Verification items for the finished model (mm, model axes). Face numbers are marked on the shaded views. Round coordinates to 2 decimals unless told otherwise and drop trailing zeros. Order: outer loops, then holes, each group sorted by start corner. A loop starts at its lowest first (then second) coordinate and runs counter-clockwise, first axis right, second up. Notation, with made-up numbers: M 29,73.5 L 76,73.5 A16 cw 76,103.5 Z; hole C -9.75,80 d1. An arc over 180 degrees is marked long. Use one line per item in the form item = value. Start each with the question number.
Item 1: Thickness scan on probe 1 along X at (y, z) = (3.6, 21); probe 2 along Y at (x, z) = (8, 19); probe 3 along X at (y, z) = (2.3, 6.5). Record the ranges inside material, lowest first. Write a range as [from, to].
Item 2: Release check for a two-part mould opening along X. For the marked faces 1, 2 and 3 record: +X half, -X half, draft (parallel to the pull), parting line (faces both ways), or undercut.
Item 3: Cross-section at A-A on y = 3.9. Enter the section's corners in (x, z), then the cut area to 3 significant figures.
Item 4: Cross-section at C-C on x = 7.25. Enter the section's corners in (y, z).
Item 5: Cross-section at D-D on y = 5.45. Enter the section's corners in (x, z).
Item 6: Cross-section at B-B on z = 14.5. Enter the section's corners in (x, y), then the cut area to 3 significant figures.
from build123d import *

# Parameters (mm, degrees)
EXTRUSION1_DEPTH = 35


with BuildPart() as part:
    # Esquisse1 → Extrusion1 (new body)
    with BuildSketch(Plane.XY):
        with BuildLine():
            Line((1.6, 5.8), (8.4, 5.8))
            ThreePointArc((8.4, 5.8), (9.53137085, 5.33137085), (10, 4.2))
            Line((10, 4.2), (10, 0))
            Line((10, 0), (8.9, 0))
            Line((8.9, 0), (8.9, 1.6))
            Line((8.9, 1.6), (9.45, 2.1))
            Line((9.45, 2.1), (8.9, 2.6))
            Line((8.9, 2.6), (8.9, 4.2))
            ThreePointArc((8.9, 4.2), (8.753553391, 4.553553391), (8.4, 4.7))
            Line((8.4, 4.7), (1.6, 4.7))
            ThreePointArc((1.6, 4.7), (1.246446609, 4.553553391), (1.1, 4.2))
            Line((1.1, 4.2), (1.1, 2.6))
            Line((1.1, 2.6), (0.55, 2.1))
            Line((0.55, 2.1), (1.1, 1.6))
            Line((1.1, 1.6), (1.1, 0))
            Line((1.1, 0), (0, 0))
            Line((0, 0), (0, 4.2))
            ThreePointArc((0, 4.2), (0.46862915, 5.33137085), (1.6, 5.8))
        make_face()
    extrude(amount=EXTRUSION1_DEPTH)


solid = part.part
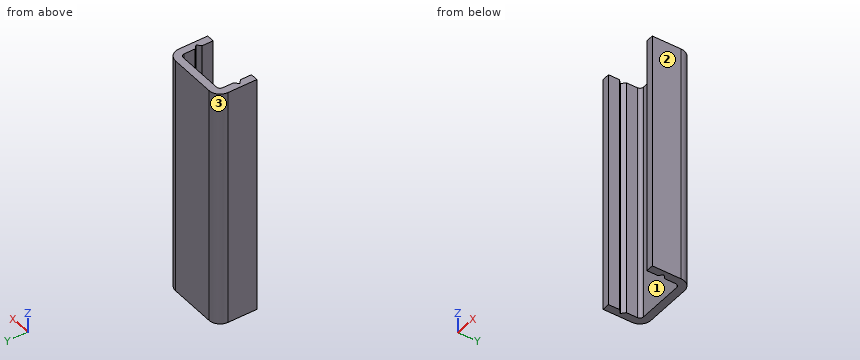
Output values:
q1.probe_1 = [0, 1.1], [8.9, 10]
q1.probe_2 = [4.7, 5.8]
q1.probe_3 = [0, 0.77], [9.23, 10]
q2.face_1 = undercut
q2.face_2 = +X half
q2.face_3 = -X half
q3.outline = M 0,0 L 1.1,0 L 1.1,35 L 0,35 Z; M 8.9,0 L 10,0 L 10,35 L 8.9,35 Z
q3.area = 77.0 mm2
q4.outline = M 4.7,0 L 5.8,0 L 5.8,35 L 4.7,35 Z
q5.outline = M 0.6,0 L 9.4,0 L 9.4,35 L 0.6,35 Z
q6.outline = M 0,0 L 1.1,0 L 1.1,1.6 L 0.55,2.1 L 1.1,2.6 L 1.1,4.2 A0.5 cw 1.6,4.7 L 8.4,4.7 A0.5 cw 8.9,4.2 L 8.9,2.6 L 9.45,2.1 L 8.9,1.6 L 8.9,0 L 10,0 L 10,4.2 A1.6 ccw 8.4,5.8 L 1.6,5.8 A1.6 ccw 0,4.2 Z
q6.area = 19.8 mm2
